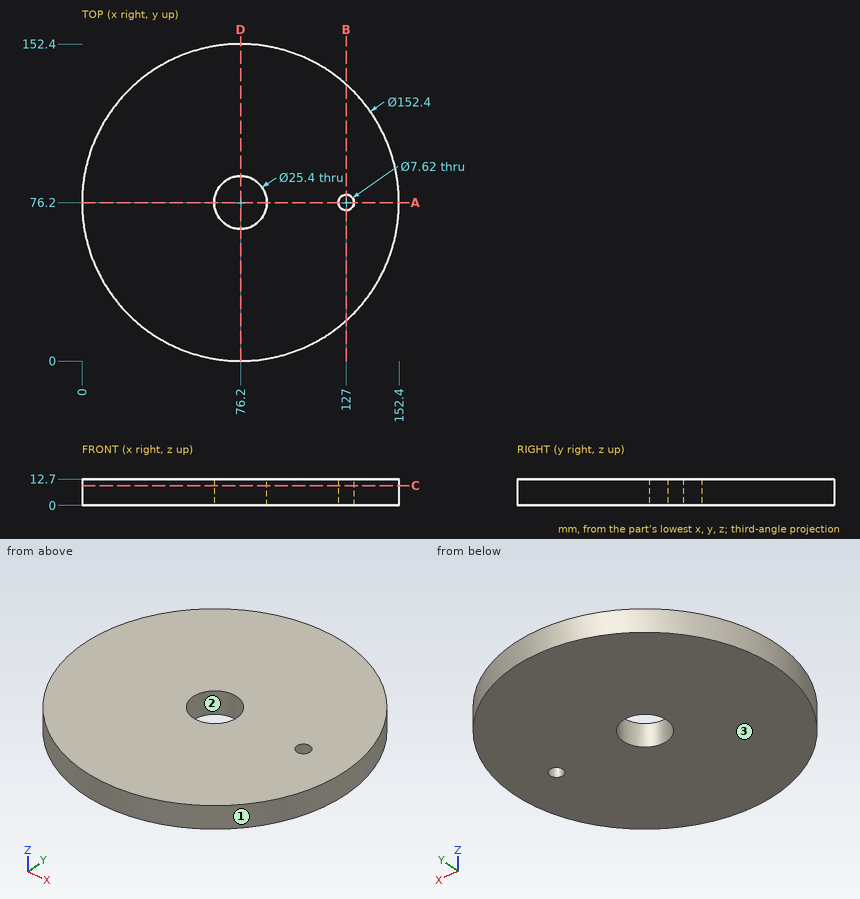
Can you work these out from the drawing? Everything is in mm from the part's minimum corner. Coordinates: 2 decimals unless noted, no trailing zeros. Order: outer loops, then holes, each group sorted by start corner. A loop starts at its lowest first (then second) coordinate and runs counter-clockwise, first axis right, second up. Notation, with made-up numbers: M 16,60.25 L 50,60.25 A24 cw 50,76.25 Z; hole C 32,7 d10. An arc over 180 degrees is marked long. Answer as CSV lines item,"result". Start each with the question number.
1. I want a section at A-A, the plane y = 76.2. Write out the boundary of the cut face in (x, z), and give its area (3 significant figures).
2. For pin 1 (12 mm diameter, centred on x = 121, y = 36, fed in from -Z); pin 2 (1 mm diameter, centred on y = 91, z = 9.5, fed in from +X); pin 3 (6 mm diameter, centred on x = 108.5, z = 6.5, fed in from +Y); pin 4 (2 mm diameter, centred on x = 33, z = 6.5, fed in from +Y), each with a flat end and sliding along its axis, tell me the tip position at first contact or that it passes through.
3. We'd pull the mould along X, two halves only. Please class the marked faces 1, 2 and 3: released by +X, released by -X, zero draft, split by the parting line, or undercut.
4. I need wall thicknesses on line 1 (Y direction, x = 76.2, z = 8); line 2 (X direction, y = 73, z = 8.5); line 3 (Y direction, x = 127, z = 6). Which ranges of each line are inside material? Lowest first, please. Write a range as [from, to].
5. I want a section at C-C, the plane z = 9.5. Write out the boundary of the cut face in (x, y), and give its area (3 significant figures).
6. I want a section at B-B, the plane x = 127. Write out the boundary of the cut face in (y, z).
7. I want a section at D-D, the plane x = 76.2. Write out the boundary of the cut face in (y, z), and give its area (3 significant figures).
Recorded:
1,outline,"M 0,0 L 63.5,0 L 63.5,12.7 L 0,12.7 Z; M 88.9,0 L 123.19,0 L 123.19,12.7 L 88.9,12.7 Z; M 130.81,0 L 152.4,0 L 152.4,12.7 L 130.81,12.7 Z"
1,area,"1,520 mm2"
2,pin 1,"stops at z = 0"
2,pin 2,"stops at x = 151.05"
2,pin 3,"stops at y = 146.54"
2,pin 4,"stops at y = 139.65"
3,face 1,"split by the parting line"
3,face 2,"undercut"
3,face 3,"zero draft"
4,line 1,"y = [0, 63.5], [88.9, 152.4]"
4,line 2,"x = [0.07, 63.91], [88.49, 124.93], [129.07, 152.33]"
4,line 3,"y = [19.4, 72.39], [80.01, 133]"
5,outline,"C 76.2,76.2 d152.4; hole C 76.2,76.2 d25.4; hole C 127,76.2 d7.62"
5,area,"17,700 mm2"
6,outline,"M 19.4,0 L 72.39,0 L 72.39,12.7 L 19.4,12.7 Z; M 80.01,0 L 133,0 L 133,12.7 L 80.01,12.7 Z"
7,outline,"M 0,0 L 63.5,0 L 63.5,12.7 L 0,12.7 Z; M 88.9,0 L 152.4,0 L 152.4,12.7 L 88.9,12.7 Z"
7,area,"1,610 mm2"
